The drawing under review shows one solid part. Ordinate dimensions are in mm from its lowest x, y, z. A direction names the side the tool comes from. Coordinates: 2 decimals unless noted, no trailing zeros. Write each loop counter-clockwise with the first axis right and the second up, starting at its lowest first coordinate (ties: lowest second). Pieces come first, ordered by that corner, then holes. Notation, with made-up numbers: (61, 46.5) - (65, 46.5) arc R22 cw to (65, 70.5) - close; hole circle Ø9 at (12, 85). An arc over 180 degrees is marked (long way). Put each result on its own line as item: value. Start each with the question number.
Item 1: Consider section A-A on z = 3. Give the boundary of the cut face in (x, y).
Item 2: To check wall thickness, follow L1, parallel to Y at x = 10, z = 7.75; L2, parallel to Y at x = 11, z = 4.25; L3, parallel to X at y = 9.25, z = 10.75 (1 decimal). State the ranges of each line that lie inside material, in increasing order. Write a range as [from, to].
Item 3: For pin 1 (1 mm diameter, centred on y = 12.5, z = 9.5, fed in from -X); pin 2 (4 mm diameter, centred on y = 17, z = 10, fed in from -X) (1 decimal); pin 3 (6 mm diameter, centred on x = 16, z = 7, fed in from +Y), all flat-tipped, find the tip position at first contact; note any pin that passes through.
Item 4: Machinability: for the marked faces 1 and 2, which of the approach directions +Z, -Z, +X, -X, +Y, -Y give a long, thin tool a straight path to every point of the face, cutting with its end or side? Answer none if there is none.
Item 5: Consider section B-B on z = 10.5. Give the boundary of the cut face in (x, y), then the cut area to 3 significant figures.
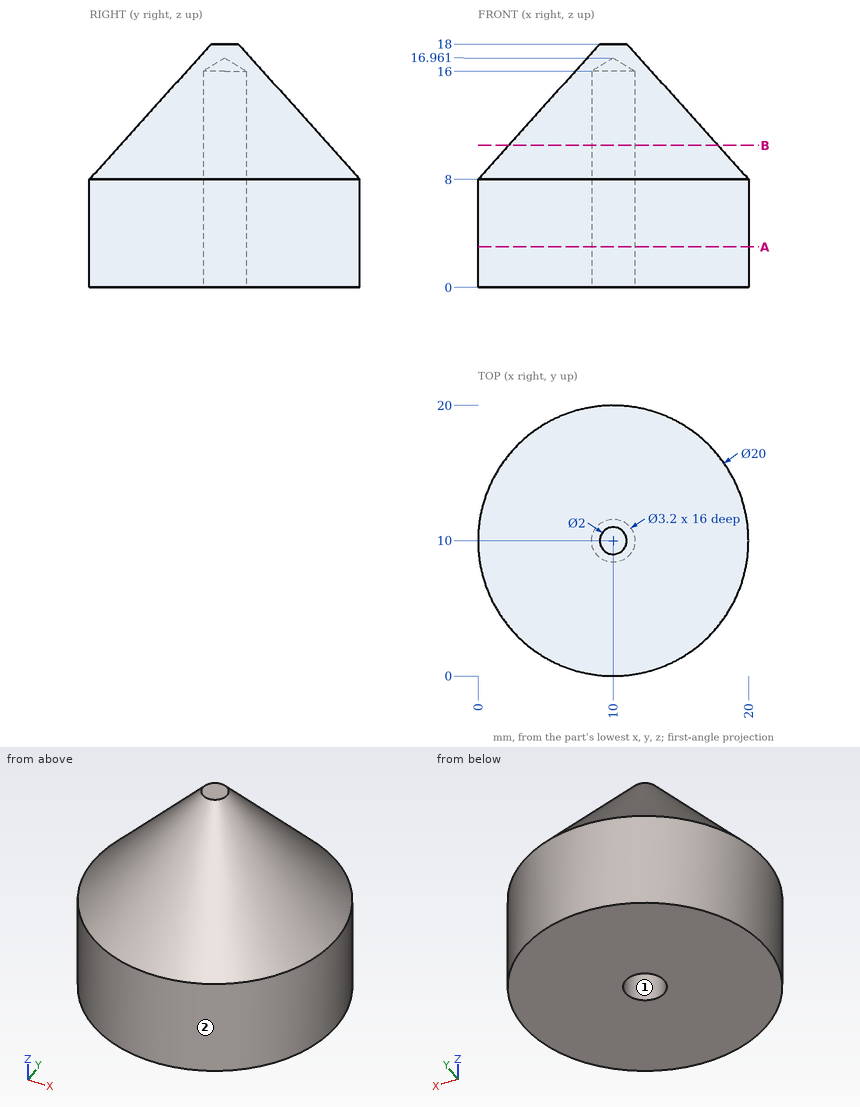
Report:
1. outline: circle Ø20 at (10, 10); hole circle Ø3.2 at (10, 10)
2. L1: [0, 8.4], [11.6, 20]
2. L2: [0.05, 8.75], [11.25, 19.95]
2. L3: [2.5, 8.6], [11.4, 17.5]
3. pin 1: x = 1.23
3. pin 2: x = 2.3
3. pin 3: y = 19.54
4. face 1: -Z
4. face 2: +Z, -Z
5. outline: circle Ø15.5 at (10, 10); hole circle Ø3.2 at (10, 10)
5. area: 181 mm²
